Could you check a few things on this model? Use its own coordinates, in mm. Face numbers are marked on the shaded views. A direction names the side the tool comes from. Round coordinates to 2 decimals unless told otherwise and drop trailing zeros. Order: outer loops, then holes, each group sorted by start corner. A loop starts at its lowest first (then second) coordinate and runs counter-clockwise, first axis right, second up.
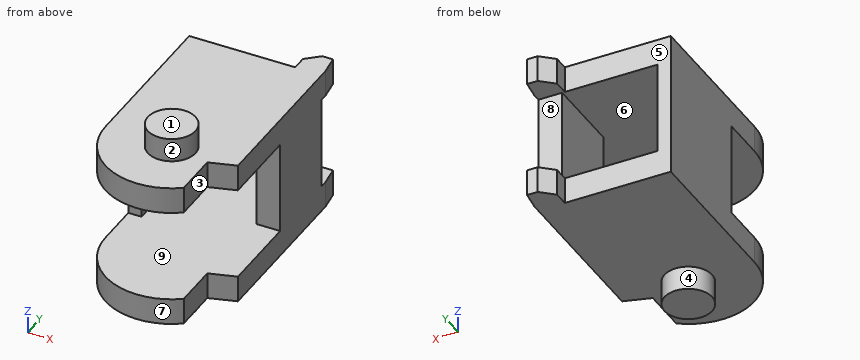
Autodesk Inventor part; units mm, degrees
ref_plane "YZ Plane" through (0, 0, 0) normal (1, 0, 0) x (0, 1, 0)
ref_plane "XZ Plane" through (0, 0, 0) normal (0, 1, 0) x (-1, 0, 0)
ref_plane "XY Plane" through (0, 0, 0) normal (0, 0, 1) x (1, 0, 0)
sketch "Skizze1" plane through (0, 0, 0) normal (0, 0, 1) x (1, 0, 0)
  arc A0 (5, -17) -> (-5, -17) centre (0, -17) ccw construction
  arc A1 (-5, -17) -> (3, -21) centre (0, -17) ccw
  circle A2 centre (0, -17) radius 1.75 construction
  line L0 (0, -22) -> (0, -4.9) construction
  line L1 (5, -17) -> (5, -4.9)
  line L2 (3, -4.9) -> (-5, -4.9)
  line L3 (-5, -4.9) -> (-5, -17)
  line L4 (0, -17) -> (3, -17) construction
  line L5 (3, -17.6027) -> (3, -21)
  line L6 (3, -17) -> (5, -17) construction
  line L7 (5, -17) -> (3, -17.6027)
  line L8 (3, -4.9) -> (3, -3.7947)
  line L9 (4, -2.9) -> (4.8065, -2.9)
  line L10 (5, -4.3512) -> (5, -4.9)
  line L11 (4, -2.9) -> (3, -3.7947)
  line L12 (4.8065, -2.9) -> (5, -4.3512)
  point P0 (0, 0)
  dimension "d0" = 3.5
  dimension "d1" = 17.1
  dimension "d2" = 3
extrude "Extrusion1" add sketch "Skizze1" against normal blind 2
sketch "Skizze2" plane through (0, 0, 0) normal (0, 0, 1) x (1, 0, 0)
  arc A0 (-5, -17) -> (3, -21) centre (0, -17) ccw
  circle A1 centre (0, -17) radius 1.8
  point P0 (0, 0)
  dimension "d7" = 3.6
extrude "Extrusion2" add sketch "Skizze2" along normal blind 1.8
sketch "Skizze4" plane through (0, 0, -2) normal (0, 0, -1) x (-1, 0, 0)
  line L0 (-5, -4.3512) -> (-5, -17) construction
  line L1 (-5, -17) -> (-3, -17.6027) construction
  line L2 (-3, -17.6027) -> (-3, -21) construction
  arc A0 (-3, -21) -> (5, -17) centre (0, -17) ccw construction
  line L3 (5, -17) -> (5, -4.9) construction
  line L4 (5, -4.9) -> (-3, -4.9) construction
  line L5 (-3, -4.9) -> (-3, -3.7947) construction
  line L6 (-3, -3.7947) -> (-4, -2.9) construction
  line L7 (-4, -2.9) -> (-4.8065, -2.9) construction
  line L8 (-4.8065, -2.9) -> (-5, -4.3512) construction
  line L9 (-5, -4.3512) -> (-5, -17) construction
  line L10 (-5, -4.9) -> (-3.2, -4.9)
  line L11 (-3.2, -4.9) -> (-3.2, -10.9)
  line L12 (-3.2, -10.9) -> (-5, -10.9)
  line L13 (-5, -10.9) -> (-5, -4.9)
  line L14 (-3, -4.9) -> (5, -4.9) construction
  line L15 (5, -4.9) -> (4, -4.9)
  line L16 (4, -4.9) -> (4, -13.7)
  line L17 (4, -13.7) -> (5, -13.7)
  line L18 (5, -13.7) -> (5, -4.9)
  point P0 (0, 0)
  dimension "d10" = 1.8
  dimension "d11" = 6
  dimension "d12" = 1
  dimension "d13" = 8.8
extrude "Extrusion3" add sketch "Skizze4" along normal blind 3.5
mirror "Spiegeln3" about plane through (4.1, -7.9, -5.5) normal (0, 0, -1) of "Extrusion2", "Extrusion1", "Extrusion3"
properties part number "chain_elmt_2"
Q1. Imagine slicing it at C-C, the plane y = -8.25. Please give me the cut outline in (x, z).
Q2. For the marked faces 1, 2, 3, 4 and 5, which set-ups out of +Z, -Z, +X, -X, +Y, -Y let a thin tool reach every point of the face, with its end or its side?
Q3. We'd pull the mould along X, two halves only. Please class the marked faces 6, 7, 8 and 9: released by +X, released by -X, zero draft, split by the parting line, or undercut.
Q4. Imagine slicing it at B-B, the plane z = -3.75. Please give me the cut outline in (x, y), then the cut area to 3 significant figures.
Q5. Imagine slicing it at A-A, the plane x = 0. Please give me the cut outline in (y, z), then the cut area to 3 significant figures.
Q6. For P1, Ø1.6, axis at y = -19.5, z = -10.5, coming from the +X side; P2, Ø3, axis at x = 2.5, z = -5.5, coming from the +Y side; P3, Ø4, axis at x = 1, z = -6, coming from the +Y side (3 decimals); P4, Ø0.9, axis at x = 4, z = -5.5, coming from the -Y side, each with a flat end and sliding along its axis, tell me the tip position at first contact or that it passes through.
Q7. I need wall thicknesses on L1, parallel to Z at x = -0.75, y = -10.25; L2, parallel to X at y = -8, z = -4; L3, parallel to Z at x = -1.5, y = -16.25. Which ranges of each line are inside material? Lowest first, please.
Q8. Imagine slicing it at D-D, the plane y = -14. Please give me the cut outline in (x, z), then the cut area to 3 significant figures.
Filled in:
1. outline: (-5, -11) - (5, -11) - (5, 0) - (-5, 0) - close; hole (-4, -9) - (3.2, -9) - (3.2, -2) - (-4, -2) - close
2. face 1: +Z, +X, -X, +Y, -Y
2. face 2: +Z
2. face 3: +Z, -Z, +X, -Y
2. face 4: -Z
2. face 5: +Z, -Z, -X, +Y
3. face 6: undercut
3. face 7: split by the parting line
3. face 8: zero draft
3. face 9: undercut
4. outline: (-5, -13.7) - (-4, -13.7) - (-4, -4.9) - (-5, -4.9) - close; (3.2, -10.9) - (5, -10.9) - (5, -4.9) - (3.2, -4.9) - close
4. area: 19.6 mm2
5. outline: (-22, -11) - (-18.8, -11) - (-18.8, -12.8) - (-15.2, -12.8) - (-15.2, -11) - (-4.9, -11) - (-4.9, -9) - (-22, -9) - close; (-22, -2) - (-4.9, -2) - (-4.9, 0) - (-15.2, 0) - (-15.2, 1.8) - (-18.8, 1.8) - (-18.8, 0) - (-22, 0) - close
5. area: 81.4 mm2
6. P1: stops at x = 3
6. P2: stops at y = -4.9
6. P3: passes through
6. P4: stops at y = -10.9
7. L1: z = -11 to -9, -2 to 0
7. L2: x = -5 to -4, 3.2 to 5
7. L3: z = -12.8 to -9, -2 to 1.8
8. outline: (-5, -11) - (5, -11) - (5, -9) - (-5, -9) - close; (-5, -2) - (5, -2) - (5, 0) - (-5, 0) - close
8. area: 40.0 mm2
